from build123d import *

# Parameters (mm, degrees)
SCHIZZO1_W                   = 42.3
SCHIZZO1_H                   = 42.3
ESTRUSIONE_ESTRUSIONE1_DEPTH = 6
FORO_PER_VITE_M3_1_OUTLINE_R = 1.7
FORO_PER_VITE_M3_1_DEPTH     = 6
ESTRUSIONE_ESTRUSIONE2_DEPTH = 42.3
ESTRUSIONE_ESTRUSIONE4_DEPTH = 42.3
RACCORDO1_R                  = 50


# Read off the part's stored shape, not the designer's step: Foro per Vite M3-1, Foro per Vite M3-2
with BuildPart() as part:
    # Schizzo1 → Estrusione-Estrusione1 (new body)
    with BuildSketch(Plane.XY):
        with Locations((-21.15, 21.15)):
            Rectangle(SCHIZZO1_W, SCHIZZO1_H)
    extrude(amount=ESTRUSIONE_ESTRUSIONE1_DEPTH)

    # Foro per Vite M3-1 outline → Foro per Vite M3-1 (cut)
    with BuildSketch(Plane.XY):
        with Locations((-5.65, 36.65)):
            Circle(FORO_PER_VITE_M3_1_OUTLINE_R)
        with Locations((-36.65, 5.65)):
            Circle(FORO_PER_VITE_M3_1_OUTLINE_R)
        with Locations((-5.65, 5.65)):
            Circle(FORO_PER_VITE_M3_1_OUTLINE_R)
        with Locations((-36.65, 36.65)):
            Circle(FORO_PER_VITE_M3_1_OUTLINE_R)
    extrude(amount=FORO_PER_VITE_M3_1_DEPTH, mode=Mode.SUBTRACT)

    # Schizzo4 → Estrusione-Estrusione2 (add)
    with BuildSketch(Plane.ZY.offset(42.3)):
        Polygon((6, 0), (8, 0), (56, 57.05), (20.410166521, 57.05), (8, 42.3), (6, 42.3), align=None)
    extrude(amount=-ESTRUSIONE_ESTRUSIONE2_DEPTH)

    # Foro per Vite M3-2 outline → Foro per Vite M3-2 (revolve, cut)
    with BuildSketch(Plane(origin=(-6.23, 0, 24.860166521), x_dir=(1, 0, 0), z_dir=(0, 0, 1))):
        Polygon((0, 57.05), (0, 52.028536948), (1.7, 53.05), (1.7, 57.05), align=None)
    revolve(axis=Axis((-6.23, 0, 24.860166521), (0, 1, 0)), mode=Mode.SUBTRACT)

    # Foro per Vite M3-2 2 outline → Foro per Vite M3-2 2 (revolve, cut)
    with BuildSketch(Plane(origin=(-36.53, 0, 43.920166521), x_dir=(1, 0, 0), z_dir=(0, 0, 1))):
        Polygon((0, 57.05), (0, 52.028536948), (1.7, 53.05), (1.7, 57.05), align=None)
    revolve(axis=Axis((-36.53, 0, 43.920166521), (0, 1, 0)), mode=Mode.SUBTRACT)

    # Foro per Vite M3-2 3 outline → Foro per Vite M3-2 3 (revolve, cut)
    with BuildSketch(Plane(origin=(-6.23, 0, 43.920166521), x_dir=(1, 0, 0), z_dir=(0, 0, 1))):
        Polygon((0, 57.05), (0, 52.028536948), (1.7, 53.05), (1.7, 57.05), align=None)
    revolve(axis=Axis((-6.23, 0, 43.920166521), (0, 1, 0)), mode=Mode.SUBTRACT)

    # Foro per Vite M3-2 4 outline → Foro per Vite M3-2 4 (revolve, cut)
    with BuildSketch(Plane(origin=(-36.53, 0, 24.860166521), x_dir=(1, 0, 0), z_dir=(0, 0, 1))):
        Polygon((0, 57.05), (0, 52.028536948), (1.7, 53.05), (1.7, 57.05), align=None)
    revolve(axis=Axis((-36.53, 0, 24.860166521), (0, 1, 0)), mode=Mode.SUBTRACT)

    # Schizzo8 → Estrusione-Estrusione4 (add)
    with BuildSketch(Plane(origin=(0, 0, 0), x_dir=(0, 0, -1), z_dir=(1, 0, 0))):
        Polygon((-8, -15.85), (67, -15.85), (67, -11.85), (32, -11.85), (32, 0), (-8, 0), align=None)
    extrude(amount=-ESTRUSIONE_ESTRUSIONE4_DEPTH)

    # Raccordo1
    # the kernel refuses this fillet: 50 mm, written as the material it adds along each edge
    with BuildSketch(Plane(origin=(-42.3, 0, 8), x_dir=(0, 0.7651893786180985, 0.6438052615892854), z_dir=(1, 0, 0))) as raccordo1_piece_1:
        with BuildLine():
            CenterArc((18.14225095, 50), RACCORDO1_R, 232.741645316, 37.258354684)
            Line((-12.128251651, 10.204313396), (-12.733661703, 9.408399664))
            ThreePointArc((-12.733661703, 9.408399664), (-6.707931087, 4.336967319), (-0.643805262, -0.765189379))
            Line((-0.643805262, -0.765189379), (0, -1))
            Line((0, -1), (18.14225095, -1))
            Line((18.14225095, -1), (18.14225095, 0))
        make_face()
    extrude(amount=42.3)


solid = part.part
Here's how the part is built. I have some questions about the finished solid (model axes, mm). A direction names the side the tool comes from. Give positions to 0.01 mm unless a question says otherwise; leave off trailing zeros. Write each loop counter-clockwise with the first axis right and the second up, starting at its lowest first coordinate (ties: lowest second). Pieces come first, ordered by that corner, then holes. Notation, with made-up numbers: (41, -34.75) -> (46, -34.75) arc R25 cw to (46, -16.75) -> close; hole circle Ø2 at (-16, 74). An arc over 180 degrees is marked (long way). Use one line per item in the form item = value. Start each with the question number.
1. Imagine slicing it at A-A on x = -11. List the corners of the cut face in (y, z) for me.
2. If I drill on L1, parallel to Y at x = -5, z = 3; L2, parallel to X at y = 36, z = 1; L3, parallel to Y at x = -2, z = -40, over which ranges is the centre line in solid material (lowest first)?
3. Imagine slicing it at B-B on y = 36.65. List the corners of the cut face in (x, z) for me, plus the area to 3 significant figures.
4. Thinking about a two-plate mould opening in Z: for faces 1 (the face through (-21, 21, 0)), 2 (the face through (-6.268, 52.206, 43.627)), 3 (the face through (-21, 0, -16)), which applies, +Z half, -Z half, draft (parallel to the pull), parting line (faces both ways), or undercut?
5. Will these pins go through, and if not, where does the flat tip stop? pin 1 Ø3 at (x, z) = (-36.53, 43.92) entering from -Y; pin 2 Ø4 at (x, y) = (-36.65, 5.65) entering from -Z; pin 3 Ø2 at (x, y) = (-36.65, 36.65) entering from +Z.
6. Imagine slicing it at C-C on z = -4. List the corners of the cut face in (x, y) for me, plus the area to 3 significant figures.
7. Imagine slicing it at D-D on y = 5.65. List the corners of the cut face in (x, z) for me.
8. On a 3-axis mill with a long thin cutter (end or side, diameter ignored), from which of +Z, -Z, +X, -X, +Y, -Y can I reach the whole of each face in a straight line? I mean faces 4 (the face through (-21, 57.05, 38)), 5 (the face through (-6, 37, 6)), 6 (the face through (-6.6, 55.08, 26.52)). Say none if no direction works.
Entries:
q1.outline = (-15.85, -67) -> (-11.85, -67) -> (-11.85, -32) -> (0, -32) -> (0, 0) -> (42.3, 0) -> (42.3, 8) -> (57.05, 20.41) -> (57.05, 56) -> (13.88, 19.68) arc R50 cw to (-15.85, 8) -> close
q2.L1 = -15.85 to 4.08, 7.22 to 35.08, 38.22 to 42.3
q2.L2 = -42.3 to -38.22, -35.08 to -7.22, -4.08 to 0
q2.L3 = -15.85 to -11.85
q3.outline = (-42.3, 0) -> (-38.35, 0) -> (-38.35, 6) -> (-34.95, 6) -> (-34.95, 0) -> (-7.35, 0) -> (-7.35, 6) -> (-3.95, 6) -> (-3.95, 0) -> (0, 0) -> (0, 38.84) -> (-42.3, 38.84) -> close
q3.area = 1,600 mm²
q4.face_1 = -Z half
q4.face_2 = undercut
q4.face_3 = draft
q5.pin_1 = 40.91
q5.pin_2 = 0
q5.pin_3 = 39.68
q6.outline = (-42.3, -15.85) -> (0, -15.85) -> (0, 0) -> (-42.3, 0) -> close
q6.area = 670 mm²
q7.outline = (-42.3, 0) -> (-38.35, 0) -> (-38.35, 6) -> (-34.95, 6) -> (-34.95, 0) -> (-7.35, 0) -> (-7.35, 6) -> (-3.95, 6) -> (-3.95, 0) -> (0, 0) -> (0, 14.05) -> (-42.3, 14.05) -> close
q8.face_4 = +Z, -Z, +X, -X, +Y
q8.face_5 = -Z
q8.face_6 = +Y
